Input: part model. Units: mm. Frame: model coordinates. A direction names the side the tool comes from. Give positions to 0.01 mm unless a question says otherwise; leave off trailing zeros. Order: outer loops, then holes, each group sorted by start corner. A loop starts at its lowest first (then second) coordinate and runs counter-clockwise, first axis right, second up. Notation, with made-up numbers: M 30,77.5 L 45,77.5 A12 cw 45,86.5 Z; hole C 63.5,54 d4. An arc over 180 degrees is marked long. Use a Markdown table: item, result.
from build123d import *

# Parameters (mm, degrees)
SKETCH2_R           = 38.1
BOSS_EXTRUDE5_DEPTH = 4.7625
SKETCH2_3_R         = 2.38125
CUT_EXTRUDE3_DEPTH  = 55.091601994


with BuildPart() as part:
    # Sketch2 → Boss-Extrude5 (new body)
    with BuildSketch(Plane(origin=(0, 0, 0), x_dir=(0, 0, -1), z_dir=(1, 0, 0))):
        with Locations(Location((0, 0, 0), (0, 0, 180))):
            Circle(SKETCH2_R)
    extrude(amount=BOSS_EXTRUDE5_DEPTH)

    # Sketch2_3 → Cut-Extrude3 (cut, through all)
    with BuildSketch(Plane(origin=(0, 0, 0), x_dir=(0, 0, -1), z_dir=(1, 0, 0))):
        with BuildLine():
            Line((21.253442374, -18.136559411), (0, -5.865878735))
            Line((0, -5.865878735), (-21.253442374, -18.136559411))
            ThreePointArc((-21.253442374, -18.136559411), (0, -27.94), (21.253442374, -18.136559411))
        make_face()
        with BuildLine():
            Line((-26.333442374, -9.337741308), (-5.08, 2.932939367))
            Line((-5.08, 2.932939367), (-5.08, 27.474300719))
            ThreePointArc((-5.08, 27.474300719), (-24.196749782, 13.97), (-26.333442374, -9.337741308))
        make_face()
        with BuildLine():
            Line((5.08, 2.932939367), (26.333442374, -9.337741308))
            ThreePointArc((26.333442374, -9.337741308), (27.535431538, -4.737468737), (27.94, 0))
            ThreePointArc((27.94, 0), (21.477648847, 17.870484045), (5.08, 27.474300719))
            Line((5.08, 27.474300719), (5.08, 2.932939367))
        make_face()
        with Locations(Location((0, 0, 0), (0, 0, 180))):
            Circle(SKETCH2_3_R)
    extrude(amount=CUT_EXTRUDE3_DEPTH, mode=Mode.SUBTRACT)


solid = part.part
1) Cut plane C-C on y = 8. Return loops of the section in (x, z).
Response values:
| item | result |
|---|---|
| outline | M 0,-37.25 L 4.76,-37.25 L 4.76,-26.77 L 0,-26.77 Z; M 0,-5.08 L 4.76,-5.08 L 4.76,5.08 L 0,5.08 Z; M 0,26.77 L 4.76,26.77 L 4.76,37.25 L 0,37.25 Z |
2) Reachability of faces 1 (the face through (2.3, -12.1, -10.8)), 2 (the face through (0, -1, 8)) from +Z, -Z, +X, -X, +Y, -Y: full face, straight path, thin tool, end or side. Return the list, or none.
Response values:
| item | result |
|---|---|
| face 1 | +X, -X |
| face 2 | +Z, -Z, -X, +Y, -Y |
3) Cut plane B-B on z = 10. Return loops of the section in (x, y), and give its area (3 significant figures).
Response values:
| item | result |
|---|---|
| outline | M 0,-36.76 L 4.76,-36.76 L 4.76,-26.09 L 0,-26.09 Z; M 0,-11.64 L 4.76,-11.64 L 4.76,0.09 L 0,0.09 Z; M 0,26.09 L 4.76,26.09 L 4.76,36.76 L 0,36.76 Z |
| area | 158 mm² |
4) Cut plane D-D on y = -7.5. Return loops of the section in (x, z).
Response values:
| item | result |
|---|---|
| outline | M 0,-37.35 L 4.76,-37.35 L 4.76,-26.91 L 0,-26.91 Z; M 0,-23.15 L 4.76,-23.15 L 4.76,-2.83 L 0,-2.83 Z; M 0,2.83 L 4.76,2.83 L 4.76,23.15 L 0,23.15 Z; M 0,26.91 L 4.76,26.91 L 4.76,37.35 L 0,37.35 Z |
5) Cut plane A-A on x = 3.95. Return loops of the section in (y, z), and give its area (3 significant figures).
Response values:
| item | result |
|---|---|
| outline | C 0,0 d76.2; hole M -18.14,-21.25 L -5.87,0 L -18.14,21.25 A27.94 ccw Z; hole M -9.34,-26.33 A27.94 ccw 27.47,-5.08 L 2.93,-5.08 Z; hole M -9.34,26.33 L 2.93,5.08 L 27.47,5.08 A27.94 ccw Z; hole C 0,0 d4.76 |
| area | 2,890 mm² |
6) Material intervals for line 1 (Y direction, x = 3.35, z = 0); line 2 (Y direction, x = 2.75, z = -10.5); line 3 (Z direction, x = 3.55, y = 23), sorted ascending. Write a range as from..to.
Response values:
| item | result |
|---|---|
| line 1 | y = -38.1..-27.94, -5.87..-2.38, 2.38..38.1 |
| line 2 | y = -36.62..-25.89, -11.93..-0.2, 25.89..36.62 |
| line 3 | z = -30.37..-15.86, -5.08..5.08, 15.86..30.37 |
7) Mould query, pull axis Z, two halves, no side actions, for faces 3 (the face through (2.348, 37.194, -8.259)), 4 (the face through (4.762, -1, 8)), 5 (the face through (2.348, 2.325, -0.516)). Classes: released by +Z, released by -Z, zero draft, split by the parting line, or undercut.
Response values:
| item | result |
|---|---|
| face 3 | split by the parting line |
| face 4 | zero draft |
| face 5 | undercut |
